Check sheet for the modelled part. Datum: model origin and axes. Units: mm. Face numbers are marked on the shaded views. Round coordinates to 2 decimals unless told otherwise and drop trailing zeros. Write each loop counter-clockwise with the first axis right and the second up, starting at its lowest first coordinate (ties: lowest second). Pieces come first, ordered by that corner, then holes.
from build123d import *

# Parameters (mm, degrees)
SKETCH1_R           = 101.6
SKETCH1_R_2         = 98.425
BOSS_EXTRUDE1_DEPTH = 406.4
CUT_EXTRUDE2_START  = 25.4
CUT_EXTRUDE2_DEPTH  = 152.4
FILLET1_R           = 12.7


with BuildPart() as part:
    # Sketch1 → Boss-Extrude1 (new body)
    with BuildSketch(Plane(origin=(0, 0, 0), x_dir=(1, 0, 0), z_dir=(0, 1, 0))):
        with Locations(Location((0, 0, 0), (0, 0, 270))):
            Circle(SKETCH1_R)
        with Locations(Location((0, 0, 0), (0, 0, 270))):
            Circle(SKETCH1_R_2, mode=Mode.SUBTRACT)
    extrude(amount=BOSS_EXTRUDE1_DEPTH)

    # Sketch3 → Cut-Extrude2 (cut)
    with BuildSketch(Plane(origin=(0, 0, 0), x_dir=(1, 0, 0), z_dir=(0, 1, 0)).offset(CUT_EXTRUDE2_START)):
        with BuildLine():
            Line((-101.352507506, -7.087257732), (-98.185241647, -6.865780928))
            ThreePointArc((-98.185241647, -6.865780928), (-71.983488082, 67.125688589), (0, 98.425))
            Line((0, 98.425), (0, 101.6))
            ThreePointArc((0, 101.6), (-74.305536085, 69.291033382), (-101.352507506, -7.087257732))
        make_face()
        with BuildLine():
            ThreePointArc((98.425, 0), (98.365042149, -3.434982963), (98.185241647, -6.865780928))
            Line((98.185241647, -6.865780928), (101.352507506, -7.087257732))
            ThreePointArc((101.352507506, -7.087257732), (101.538108025, -3.545788865), (101.6, 0))
            ThreePointArc((101.6, 0), (71.842048969, 71.842048969), (0, 101.6))
            Line((0, 101.6), (0, 98.425))
            ThreePointArc((0, 98.425), (69.596984938, 69.596984938), (98.425, 0))
        make_face()
    extrude(amount=CUT_EXTRUDE2_DEPTH, mode=Mode.SUBTRACT)

    # Fillet1
    fillet1_edges = [part.edges().sort_by_distance(p)[0] for p in [
        (99.768874577, 25.4, 6.97651933),
        (-99.768874577, 177.8, 6.97651933),
        (99.768874577, 177.8, 6.97651933),
        (-99.768874577, 25.4, 6.97651933),
    ]]
    fillet(fillet1_edges, radius=FILLET1_R)


solid = part.part
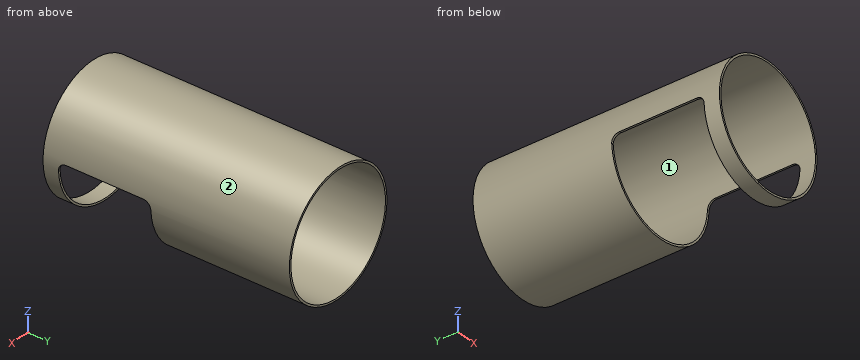
1. Scan lines: line 1 along X through (y, z) = (247, 0) (3 decimals); line 2 along Z through (x, y) = (-0.5, 370.5); line 3 along Z through (x, y) = (-32, 238). Record each from-to range of solid material in increasing order.
2. Sectioned sample at D-D, the plane x = -66.5. Enter the section's corners in (y, z), plus the area to 3 significant figures.
3. Sectioned sample at C-C, the plane z = -15. Enter the section's corners in (x, y), plus the area to 3 significant figures.
4. Sectioned sample at B-B, the plane z = 63.5. Enter the section's corners in (x, y), plus the area to 3 significant figures.
5. Sectioned sample at A-A, the plane x = 0. Enter the section's corners in (y, z) (3 decimals), plus the area to 3 significant figures.
6. Go/stop test with flat-tipped pins: pin 1 (6 mm diameter, centred on y = 189, z = -37.5, fed in from -X); pin 2 (10 mm diameter, centred on x = 39.5, y = 68.5, fed in from -Z); pin 3 (1 mm diameter, centred on y = 228, z = -24, fed in from +X). Record where each tip stops, or that it passes through.
7. Release check for a two-part mould opening along X. For the marked faces 1 and 2 record: released by +X, released by -X, zero draft, split by the parting line, or undercut.
Computed values:
1. line 1: x = -101.6 to -98.425, 98.425 to 101.6
1. line 2: z = -101.6 to -98.42, 98.42 to 101.6
1. line 3: z = -96.43 to -93.08, 93.08 to 96.43
2. outline: (0, -76.81) - (25.4, -76.81) - (25.4, -72.56) - (0, -72.56) - close; (0, 72.56) - (406.4, 72.56) - (406.4, 76.81) - (0, 76.81) - close; (177.8, -76.81) - (406.4, -76.81) - (406.4, -72.56) - (177.8, -72.56) - close
2. area: 2,810 mm2
3. outline: (-100.49, 0) - (-97.28, 0) - (-97.28, 25.4) - (-100.49, 25.4) - close; (-100.49, 177.8) - (-97.28, 177.8) - (-97.28, 406.4) - (-100.49, 406.4) - close; (97.28, 0) - (100.49, 0) - (100.49, 25.4) - (97.28, 25.4) - close; (97.28, 177.8) - (100.49, 177.8) - (100.49, 406.4) - (97.28, 406.4) - close
3. area: 1,630 mm2
4. outline: (-79.31, 0) - (-75.2, 0) - (-75.2, 406.4) - (-79.31, 406.4) - close; (75.2, 0) - (79.31, 0) - (79.31, 406.4) - (75.2, 406.4) - close
4. area: 3,340 mm2
5. outline: (0, -101.6) - (25.4, -101.6) - (25.4, -98.425) - (0, -98.425) - close; (0, 98.425) - (406.4, 98.425) - (406.4, 101.6) - (0, 101.6) - close; (177.8, -101.6) - (406.4, -101.6) - (406.4, -98.425) - (177.8, -98.425) - close
5. area: 2,100 mm2
6. pin 1: stops at x = -95.56
6. pin 2: stops at z = 87.79
6. pin 3: stops at x = 98.84
7. face 1: undercut
7. face 2: split by the parting line
